Geometry: final body of the model. Coordinates: model frame, mm. Face numbers are marked on the shaded views. A direction names the side the tool comes from. Give positions to 0.01 mm unless a question says otherwise; leave off trailing zeros. Loops run counter-clockwise (first coordinate to the right, second up) from the corner with the lowest first, then second, coordinate; pieces in that order, holes last. Notation, with made-up numbers: (75, -38.75) - (96, -38.75) arc R25 ccw to (96, -13.75) - close; hole circle Ø5 at (-26, 23). An arc over 180 degrees is marked (long way). Answer in a Markdown table with one row per item.
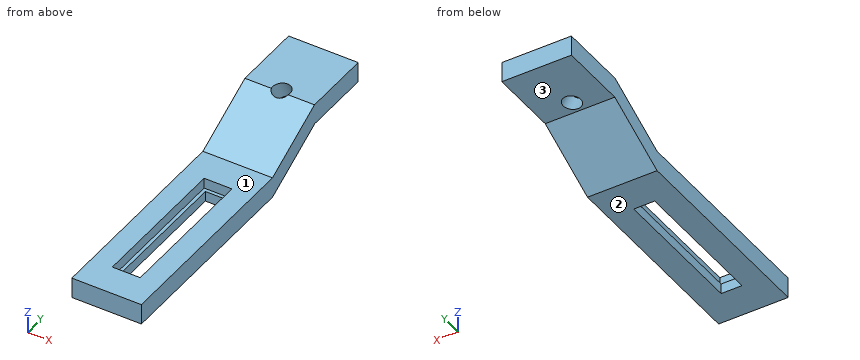
Autodesk Inventor part; units mm, degrees
ref_plane "YZ Plane" through (0, 0, 0) normal (1, 0, 0) x (0, 1, 0)
ref_plane "XZ Plane" through (0, 0, 0) normal (0, 1, 0) x (-1, 0, 0)
ref_plane "XY Plane" through (0, 0, 0) normal (0, 0, 1) x (1, 0, 0)
sketch "Эскиз1" plane through (0, 0, 0) normal (1, 0, 0) x (0, 1, 0)
  line L0 (13.9581, 11.7453) -> (25.9581, 11.7453)
  line L1 (25.9581, 11.7453) -> (25.9581, 13.7453)
  line L2 (25.9581, 13.7453) -> (13.9581, 13.7453)
  line L3 (13.9581, 13.7453) -> (13.9581, 11.7453)
  line L4 (13.9581, 11.7453) -> (13.9581, -21.2547)
  line L5 (13.9581, -21.2547) -> (25.9581, -21.2547)
  line L6 (25.9581, -21.2547) -> (25.9581, 11.7453)
  line L7 (13.9581, 11.7453) -> (13.9581, 7.7453)
  line L8 (13.9581, 7.7453) -> (25.9581, 7.7453)
  line L9 (-6.8518, -18.2547) -> (-6.8518, 11.7453)
  line L10 (-6.8518, 11.7453) -> (-15.825, 11.7453)
  line L11 (-15.825, 11.7453) -> (-15.825, 14.7104)
  line L12 (-15.825, 14.7104) -> (-5.825, 14.7104)
  line L13 (-5.825, 14.7104) -> (-5.825, 11.7453)
  line L14 (-15.825, 14.7104) -> (-25.825, 14.7104)
  line L15 (-25.825, 14.7104) -> (-25.825, 11.7453)
  line L16 (-15.825, 11.7453) -> (-25.825, 11.7453)
  line L17 (-5.825, 14.7104) -> (4.175, 14.7104)
  line L18 (4.175, 14.7104) -> (4.175, 11.7453)
  line L19 (13.9581, 7.7453) -> (23.1232, 11.7453)
  line L20 (23.1232, 11.7453) -> (18.5407, 9.7453)
  line L21 (18.5407, 9.7453) -> (19.9154, 10.3453)
  line L22 (18.5407, 9.7453) -> (17.1659, 9.1453)
  line L23 (19.9154, 10.3453) -> (15.1154, 21.3434)
  line L24 (17.1659, 9.1453) -> (12.3659, 20.1434)
  line L25 (12.3659, 20.1434) -> (15.1154, 21.3434)
  line L26 (13.9581, 11.7453) -> (13.8495, 16.7441)
  line L27 (13.8495, 16.7441) -> (4.175, 11.7453)
  line L28 (4.175, 14.7104) -> (13.7858, 19.6763)
  line L29 (13.7858, 19.6763) -> (23.7858, 19.6763)
  line L30 (23.7858, 19.6763) -> (23.7858, 16.7441)
  line L31 (23.7858, 16.7441) -> (13.8495, 16.7441)
  line L32 (4.175, 11.7453) -> (-5.825, 11.7453)
  line L33 (-5.825, 11.7453) -> (-6.8518, 11.7453)
  point P0 (0, 0)
  dimension "d0" = 12
  dimension "d1" = 2
  dimension "d2" = 33
  dimension "d3" = 4
  dimension "d4" = 10
  dimension "d5" = 10
  dimension "d6" = 10
  dimension "d7" = 10
  dimension "d8" = 1.5
  dimension "d9" = 1.5
  dimension "d10" = 12
  dimension "d11" = 12
  dimension "d12" = 5
  dimension "d13" = 10
extrude "Выдавливание1" add sketch "Эскиз1" along normal blind 5 and the other way blind 5 contours L31 L24 L28 L29 L23 | L23 L29 L30 L31 | L27 L18 L28 L24 | L32 L13 L17 L18 | L33 L10 L11 L12 L13 | L11 L16 L15 L14
sketch "Эскиз2" plane through (-5, 4.175, 14.7104) normal (0, -0.459, 0.8884) x (1, 0, 0)
  line L0 (5, 9.6975) -> (5, 12.6658)
  line L1 (5, 12.6658) -> (5, 11.1658)
  circle A0 centre (5, 11.1658) radius 1.25
  point P0 (5, -10.4618)
  dimension "d18" = 1.5
  dimension "d19" = 2.5
sketch "Эскиз3" plane through (-5, -25.825, 14.7104) normal (0, 0, 1) x (1, 0, 0)
  line L0 (0, 0) -> (10, 0)
  line L1 (5, 0) -> (5, 10)
  line L2 (5, 10) -> (0, 10)
  line L3 (0, 10) -> (0, 20)
  line L4 (0, 20) -> (10, 20)
  line L5 (10, 20) -> (10, 10)
  line L6 (10, 30) -> (10, 0)
  line L7 (5, 10) -> (10, 10)
  line L8 (5, 10) -> (3.5, 10)
  line L9 (3.5, 10) -> (3.5, 20)
  line L10 (3.5, 20) -> (3.5, 25)
  line L11 (3.5, 25) -> (6.5, 25)
  line L12 (6.5, 25) -> (6.5, 5)
  line L13 (6.5, 5) -> (3.5, 5)
  line L14 (3.5, 5) -> (3.5, 10)
  line L15 (5, 10) -> (7, 10)
  line L16 (7, 10) -> (7, 4.5)
  line L17 (7, 4.5) -> (3, 4.5)
  line L18 (3, 4.5) -> (3, 25.5)
  line L19 (3, 25.5) -> (7, 25.5)
  line L20 (7, 25.5) -> (7, 10)
  line L21 (7, 10) -> (7, 4.5)
  line L22 (7, 4.5) -> (5, 4.5)
  line L23 (5, 4.5) -> (5, 10)
  line L24 (6.5, 10) -> (5, 10)
  line L25 (5, 10) -> (5, 5)
  line L26 (5, 5) -> (6.5, 5)
  line L27 (6.5, 5) -> (6.5, 10)
  point P0 (5, 25.825)
  point P1 (5, 5)
  point P2 (5, 5)
  dimension "d22" = 10
  dimension "d23" = 10
  dimension "d24" = 1.5
  dimension "d25" = 5
  dimension "d26" = 3
  dimension "d27" = 20
  dimension "d28" = 2
  dimension "d29" = 5.5
  dimension "d30" = 4
  dimension "d31" = 21
extrude "Выдавливание3" cut sketch "Эскиз3" against normal blind 5 contours L13 L14 L2 L1 | L2 L9 L4 L12 L7 | L4 L10 L11 L12
extrude "Выдавливание4" cut sketch "Эскиз3" against normal blind 1.5 contours L17 L18 L2 L14 L13 L1 | L1 L13 L12 L7 L16 L17 | L1 L7 L12 L13 | L7 L12 L4 L20 | L18 L4 L9 L2 | L4 L12 L11 L10 L18 L19 L20
extrude "Выдавливание5" cut sketch "Эскиз3" against normal blind 3 contours L1 L7 L12 L13
extrude "Выдавливание6" cut sketch "Эскиз2" against normal blind 10
properties part number "micro_wheel_mount"
Q1. Cut plane C-C (x = 0.75). Output: boundary loops of the cut face in (y, z) (1 decimal), and give its area (3 significant figures).
Check values:
| item | result |
|---|---|
| outline | (-25.8, 11.7) - (-20.8, 11.7) - (-20.8, 13.2) - (-21.3, 13.2) - (-21.3, 14.7) - (-25.8, 14.7) - close; (-0.8, 11.7) - (4.2, 11.7) - (13.8, 16.7) - (14.6, 16.7) - (13.2, 19.4) - (4.2, 14.7) - (-0.3, 14.7) - (-0.3, 13.2) - (-0.8, 13.2) - close; (15.3, 19.7) - (16.8, 16.7) - (23.8, 16.7) - (23.8, 19.7) - close |
| area | 79.5 mm² |
Q2. Cut plane B-B (x = 4). Output: boundary loops of the cut face in (y, z) (1 decimal), and give its area (3 significant figures).
Check values:
| item | result |
|---|---|
| outline | (-25.8, 11.7) - (4.2, 11.7) - (13.8, 16.7) - (23.8, 16.7) - (23.8, 19.7) - (13.8, 19.7) - (4.2, 14.7) - (-25.8, 14.7) - close |
| area | 147 mm² |
Q3. Cut plane D-D (y = 12.5). Output: boundary loops of the cut face in (x, z), and give its area (3 significant figures).
Check values:
| item | result |
|---|---|
| outline | (-5, 16.05) - (5, 16.05) - (5, 19.01) - (-5, 19.01) - close |
| area | 29.7 mm² |
Q4. Material intervals for line 1 along X through (y, z) = (-4, 13.5); line 2 along X through (y, z) = (-9, 12.75); line 3 along Z through (x, y) = (-1.75, 0.5), sorted ascending.
Check values:
| item | result |
|---|---|
| line 1 | -5 to -2, 2 to 5 |
| line 2 | -5 to -1.5, 1.5 to 5 |
| line 3 | 11.75 to 14.71 |
Q5. Reachability of the marked faces 1, 2 and 3 from +Z, -Z, +X, -X, +Y, -Y: full face, straight path, thin tool, end or side. Return the list, or none.
Check values:
| item | result |
|---|---|
| face 1 | +Z, +X, -X, -Y |
| face 2 | -Z, +X, -X, +Y, -Y |
| face 3 | -Z, +X, -X, +Y |
Q6. Cut plane A-A (y = -2.5). Output: boundary loops of the cut face in (x, z), and give its area (3 significant figures).
Check values:
| item | result |
|---|---|
| outline | (-5, 11.75) - (-1.5, 11.75) - (-1.5, 13.21) - (-2, 13.21) - (-2, 14.71) - (-5, 14.71) - close; (1.5, 11.75) - (5, 11.75) - (5, 14.71) - (2, 14.71) - (2, 13.21) - (1.5, 13.21) - close |
| area | 19.3 mm² |
Q7. First-contact query: pin 1 (1 mm diameter, centred on x = 1, z = 15.5, fed in from -Y); pin 2 (1.6 mm diameter, centred on x = 0, z = 14, fed in from +Y); pin 3 (3 mm diameter, centred on x = -2, y = 20, fed in from -Z); pin 4 (1.2 mm diameter, centred on x = -0.5, y = -10, fed in from +Z). Flat tips, straight axial feed; report the tip coordinate or a pass-through.
Check values:
| item | result |
|---|---|
| pin 1 | y = 4.74 |
| pin 2 | y = 10.09 |
| pin 3 | z = 16.74 |
| pin 4 | through |
